Check sheet for the modelled part. Datum: model origin and axes. Units: mm. A direction names the side the tool comes from. Round coordinates to 2 decimals unless told otherwise and drop trailing zeros. Write each loop counter-clockwise with the first axis right and the second up, starting at its lowest first coordinate (ties: lowest second). Pieces come first, ordered by that corner, then holes. Notation, with made-up numbers: M 75,80 L 117,80 A21 cw 117,100 Z; hole C 54.5,43 d9. An arc over 180 degrees is marked long. One line per item, written item: value.
from build123d import *

# Parameters (mm, degrees)
SKETCH1_W                = 29
SKETCH1_H                = 29.8
SKETCH1_W_2              = 23
SKETCH1_H_2              = 23.8
SIDES_DEPTH              = 13
SKETCH2_W                = 29
SKETCH2_H                = 29.8
BASE_DEPTH               = 3
SKETCH3_W                = 29
SKETCH3_H                = 3
SERVO_WING_SLOTS_DEPTH   = 13
SKETCH4_W                = 3
SKETCH4_H                = 3.5
SERVO_WIRE_SLOT_DEPTH    = 13
SKETCH5_W                = 15
SKETCH5_H                = 3
SERVO_HEAD_OPENING_DEPTH = 13
MOUNT_REACH              = 41.538
SKETCH6_R                = 2
MOUNT_DIRECTION_2_REACH  = 41.538


with BuildPart() as part:
    # Sketch1 → sides (new body)
    with BuildSketch(Plane(origin=(0, 0, 0), x_dir=(0, 0, -1), z_dir=(1, 0, 0))):
        with Locations((11.5, 11.9)):
            Rectangle(SKETCH1_W, SKETCH1_H)
        with Locations((11.5, 11.9)):
            Rectangle(SKETCH1_W_2, SKETCH1_H_2, mode=Mode.SUBTRACT)
    extrude(amount=SIDES_DEPTH)

    # Sketch2 → base (add)
    with BuildSketch(Plane(origin=(0, 0, 0), x_dir=(0, 0, -1), z_dir=(1, 0, 0))):
        with Locations((11.5, 11.9)):
            Rectangle(SKETCH2_W, SKETCH2_H)
    extrude(amount=-BASE_DEPTH)

    # Sketch3 → servo wing slots (cut)
    with BuildSketch(Plane(origin=(0, 0, 0), x_dir=(0, 0, -1), z_dir=(1, 0, 0))):
        with Locations((11.5, 18.05)):
            Rectangle(SKETCH3_W, SKETCH3_H)
    extrude(amount=SERVO_WING_SLOTS_DEPTH, mode=Mode.SUBTRACT)

    # Sketch4 → servo wire slot (cut)
    with BuildSketch(Plane(origin=(0, 0, 0), x_dir=(0, 0, -1), z_dir=(1, 0, 0))):
        with Locations((-1.5, 5.25)):
            Rectangle(SKETCH4_W, SKETCH4_H)
    extrude(amount=SERVO_WIRE_SLOT_DEPTH, mode=Mode.SUBTRACT)

    # Sketch5 → servo head opening (cut)
    with BuildSketch(Plane(origin=(0, 0, 0), x_dir=(0, 0, -1), z_dir=(1, 0, 0))):
        with Locations((7.5, 25.3)):
            Rectangle(SKETCH5_W, SKETCH5_H)
    extrude(amount=SERVO_HEAD_OPENING_DEPTH, mode=Mode.SUBTRACT)

    # mount: up to this face of the body (flat: up to its plane)
    mount_end = Plane(part.part.faces().sort_by_distance((13, 11.775, 1.5))[0])
    # Sketch6 → mount (add, up to the picked face)
    with BuildSketch(Plane(origin=(0, 0, 0), x_dir=(0, 0, -1), z_dir=(1, 0, 0)), mode=Mode.PRIVATE) as mount_sk1:
        with BuildLine():
            Line((-6, 15.4), (-3, 15.4))
            Line((-3, 15.4), (-3, 8.4))
            Line((-3, 8.4), (-6, 8.4))
            ThreePointArc((-6, 8.4), (-9.5, 11.9), (-6, 15.4))
        make_face()
        with Locations(Location((-6, 11.9, 0), (0, 0, 180))):
            Circle(SKETCH6_R, mode=Mode.SUBTRACT)
    mount_tool1 = split(extrude(mount_sk1.sketch, amount=MOUNT_REACH, mode=Mode.PRIVATE), bisect_by=mount_end, keep=Keep.BOTH, mode=Mode.PRIVATE)
    # Sketch6 → mount (add, up to the picked face)
    with BuildSketch(Plane(origin=(0, 0, 0), x_dir=(0, 0, -1), z_dir=(1, 0, 0)), mode=Mode.PRIVATE) as mount_sk2:
        with BuildLine():
            Line((29, 15.4), (26, 15.4))
            Line((26, 15.4), (26, 8.4))
            Line((26, 8.4), (29, 8.4))
            ThreePointArc((29, 8.4), (32.5, 11.9), (29, 15.4))
        make_face()
        with Locations(Location((29, 11.9, 0), (0, 0, 180))):
            Circle(SKETCH6_R, mode=Mode.SUBTRACT)
    mount_tool2 = split(extrude(mount_sk2.sketch, amount=MOUNT_REACH, mode=Mode.PRIVATE), bisect_by=mount_end, keep=Keep.BOTH, mode=Mode.PRIVATE)
    add(mount_tool1.solids().sort_by(Axis((0, 15.304475, 4.5), (1, 0, 0)))[0])
    add(mount_tool2.solids().sort_by(Axis((0, 11.9, -32.404475), (1, 0, 0)))[0])

    # mount direction 2: up to this face of the body (flat: up to its plane)
    mount_direction_2_end = Plane(part.part.faces().sort_by_distance((-3, 11.9, -11.5))[0])
    # Sketch6 → mount direction 2 (add, up to the picked face)
    with BuildSketch(Plane(origin=(0, 0, 0), x_dir=(0, 0, -1), z_dir=(1, 0, 0)), mode=Mode.PRIVATE) as mount_direction_2_sk1:
        with BuildLine():
            Line((-6, 15.4), (-3, 15.4))
            Line((-3, 15.4), (-3, 8.4))
            Line((-3, 8.4), (-6, 8.4))
            ThreePointArc((-6, 8.4), (-9.5, 11.9), (-6, 15.4))
        make_face()
        with Locations(Location((-6, 11.9, 0), (0, 0, 180))):
            Circle(SKETCH6_R, mode=Mode.SUBTRACT)
    mount_direction_2_tool1 = split(extrude(mount_direction_2_sk1.sketch, amount=-MOUNT_DIRECTION_2_REACH, mode=Mode.PRIVATE), bisect_by=mount_direction_2_end, keep=Keep.BOTH, mode=Mode.PRIVATE)
    # Sketch6 → mount direction 2 (add, up to the picked face)
    with BuildSketch(Plane(origin=(0, 0, 0), x_dir=(0, 0, -1), z_dir=(1, 0, 0)), mode=Mode.PRIVATE) as mount_direction_2_sk2:
        with BuildLine():
            Line((29, 15.4), (26, 15.4))
            Line((26, 15.4), (26, 8.4))
            Line((26, 8.4), (29, 8.4))
            ThreePointArc((29, 8.4), (32.5, 11.9), (29, 15.4))
        make_face()
        with Locations(Location((29, 11.9, 0), (0, 0, 180))):
            Circle(SKETCH6_R, mode=Mode.SUBTRACT)
    mount_direction_2_tool2 = split(extrude(mount_direction_2_sk2.sketch, amount=-MOUNT_DIRECTION_2_REACH, mode=Mode.PRIVATE), bisect_by=mount_direction_2_end, keep=Keep.BOTH, mode=Mode.PRIVATE)
    add(mount_direction_2_tool1.solids().sort_by(Axis((0, 15.304475, 4.5), (-1, 0, 0)))[0])
    add(mount_direction_2_tool2.solids().sort_by(Axis((0, 11.9, -32.404475), (-1, 0, 0)))[0])


solid = part.part
Q1. Scan lines: line 1 (Z direction, x = 0.75, y = 11.9); line 2 (Y direction, x = 1.25, z = 1); line 3 (Y direction, x = 0.5, z = -21). Record each from-to range of solid material in increasing order. Write a range as [from, to].
Completed:
line 1: [-32.5, -31], [-27, -23], [0, 4], [8, 9.5]
line 2: [-3, 3.5], [7, 16.55], [19.55, 26.8]
line 3: [-3, 0], [23.8, 26.8]
Q2. Sectioned sample at B-B on y = 11.9. Enter the section's corners in (x, z).
Completed:
outline: M -3,-32.5 L 13,-32.5 L 13,-31 L -3,-31 Z; M -3,-27 L 13,-27 L 13,-23 L 0,-23 L 0,0 L 13,0 L 13,4 L -3,4 Z; M -3,8 L 13,8 L 13,9.5 L -3,9.5 Z
Q3. Sectioned sample at A-A on x = 3.25. State how many separate pieces and enclosed holes the cut face has, and give its area (3 significant figures).
Completed:
separate pieces: 4
enclosed holes: 2
area: 299 mm^2
Q4. Sectioned sample at C-C on z = -10. Enter the section's corners in (x, y), and give its area (3 significant figures).
Completed:
outline: M -3,-3 L 13,-3 L 13,0 L 0,0 L 0,26.8 L -3,26.8 Z
area: 128 mm^2
Q5. Sectioned sample at D-D on y = 18.75. Enter the section's corners in (x, z).
Completed:
outline: M -3,-26 L 0,-26 L 0,3 L -3,3 Z
Q6. Depth check by flat-ended pin: P1, Ø1.5, axis at x = 7.5, z = -27.5, coming from the -Y side; P2, Ø5, axis at x = 1.5, y = 22, coming from the -Z side; P3, Ø2, axis at x = 8.5, y = 0.5, coming from the +Z side. Enter the tip coordinate at first touch or a pass-through.
Completed:
P1: y = 8.4
P2: z = -26
P3: z = 3
Q7. Draft check along Y on faces 6 (the flat face through (6, 7, 2)), 7 (the flat face through (5, 8.4, 4)), 8 (the flat face through (5, 1, 3)). Enter one of: pulls with the +Y half, pulls with the -Y half, needs draft (parallel to the pull), parting line crosses it, or undercut.
Completed:
face 6: undercut
face 7: pulls with the -Y half
face 8: needs draft
Q8. Access from +Z, -Z, +X, -X, +Y, -Y to the whole of each face (thin tool, end or side, straight path). Record for faces 1 (the flat face through (6, 16.55, 2)), 2 (the flat face through (6, 3.5, 2)), 3 (the flat face through (5, 8.4, -27)), 4 (the flat face through (6, 23.8, -19)), 5 (the flat face through (5, 15.4, 5)).
Completed:
face 1: +Z, -Z, +X
face 2: +Z, +X
face 3: -Z, +X, -X, -Y
face 4: +X
face 5: +Z, +X, -X, +Y
